```python
from build123d import *

# Parameters (mm, degrees)
F3_D    = 29
F4_SIZE = 0.5


with BuildPart() as f1:
    # F0 (on Front) → F1 (revolve)
    with BuildSketch(Plane.XZ):
        Polygon((0, -15.5), (0, 0), (-19.5, 0), (-16.5, -3), (-16.5, -15.5), align=None)
    revolve(axis=Axis((0, 0, -7.75), (0, 0, 1)))

    # F3 (through all)
    with Locations(Plane.XY):
        with Locations((0, 0)):
            Hole(F3_D / 2)

    # F4
    f4_edges = [f1.edges().sort_by_distance(p)[0] for p in [
        (16.5, 0, -15.5),
    ]]
    chamfer(f4_edges, length=F4_SIZE)


solid = f1.part
```
Source: CAD feature listing. Evaluate the final solid. Frame: model axes, mm. Coordinates: 2 decimals unless noted, no trailing zeros. Loops run counter-clockwise (first coordinate to the right, second up) from the corner with the lowest first, then second, coordinate; pieces in that order, holes last. Notation, with made-up numbers: M 2.25,-31.5 L 13.25,-31.5 A20 ccw 13.25,-14.5 Z; hole C 78.25,44.25 d7. An arc over 180 degrees is marked long. Use a Markdown table: item, result. Add a question column.
Q1. Section query C-C, the plane z = -9.25. Return loops of the section in (x, y), and give its area (3 significant figures).
Q2. Material intervals for L1, parallel to Y at x = 0, z = -9.25; L2, parallel to Y at x = 2, z = -8.25; L3, parallel to X at y = -13, z = -2, sorted ascending.
Q3. Draft query along Y for faces 1 (the cylindrical face through (-6.691, -12.864, -7.858)), 2 (the cylindrical face through (-15.24, 6.32, -9.08)), 3 (the flat face through (0, -15, 0)). Return one class per face: pulls with the +Y half, pulls with the -Y half, needs draft (parallel to the pull), parting line crosses it, or undercut.
Q4. Section query A-A, the plane y = 0. Return loops of the section in (x, z), and give its area (4 significant figures).
Q5. First-contact query: pin 1 (5 mm diameter, centred on y = 4.5, z = -6.5, fed in from -X); pin 2 (6 mm diameter, centred on x = -11.5, z = -5, fed in from +Y); pin 3 (2 mm diameter, centred on y = -6.5, z = -11, fed in from +X). Flat tips, straight axial feed; report the tip coordinate or a pass-through.
Result:
| question | item | result |
|---|---|---|
| 1 | outline | C 0,0 d33; hole C 0,0 d29 |
| 1 | area | 195 mm2 |
| 2 | L1 | y = -16.5 to -14.5, 14.5 to 16.5 |
| 2 | L2 | y = -16.38 to -14.36, 14.36 to 16.38 |
| 2 | L3 | x = -11.72 to -6.42, 6.42 to 11.72 |
| 3 | face 1 | undercut |
| 3 | face 2 | parting line crosses it |
| 3 | face 3 | needs draft |
| 4 | outline | M -19.5,0 L -16.5,-3 L -16.5,-15 L -16,-15.5 L -14.5,-15.5 L -14.5,0 Z; M 14.5,-15.5 L 16,-15.5 L 16.5,-15 L 16.5,-3 L 19.5,0 L 14.5,0 Z |
| 4 | area | 70.75 mm2 |
| 5 | pin 1 | stops at x = -16.38 |
| 5 | pin 2 | stops at y = 14.14 |
| 5 | pin 3 | stops at x = 15.56 |
